Can you work these out from the drawing? Everything is in mm from the part's minimum corner. Round coordinates to 2 decimals unless told otherwise and drop trailing zeros. Loops run counter-clockwise (first coordinate to the right, second up) from the corner with the lowest first, then second, coordinate; pieces in that order, holes last. Notation, with made-up numbers: M -15,-0.5 L 33,-0.5 A24 cw 33,32.5 Z; hole C -14,80.5 d7. An arc over 180 degrees is marked long. Use a Markdown table: item, result.
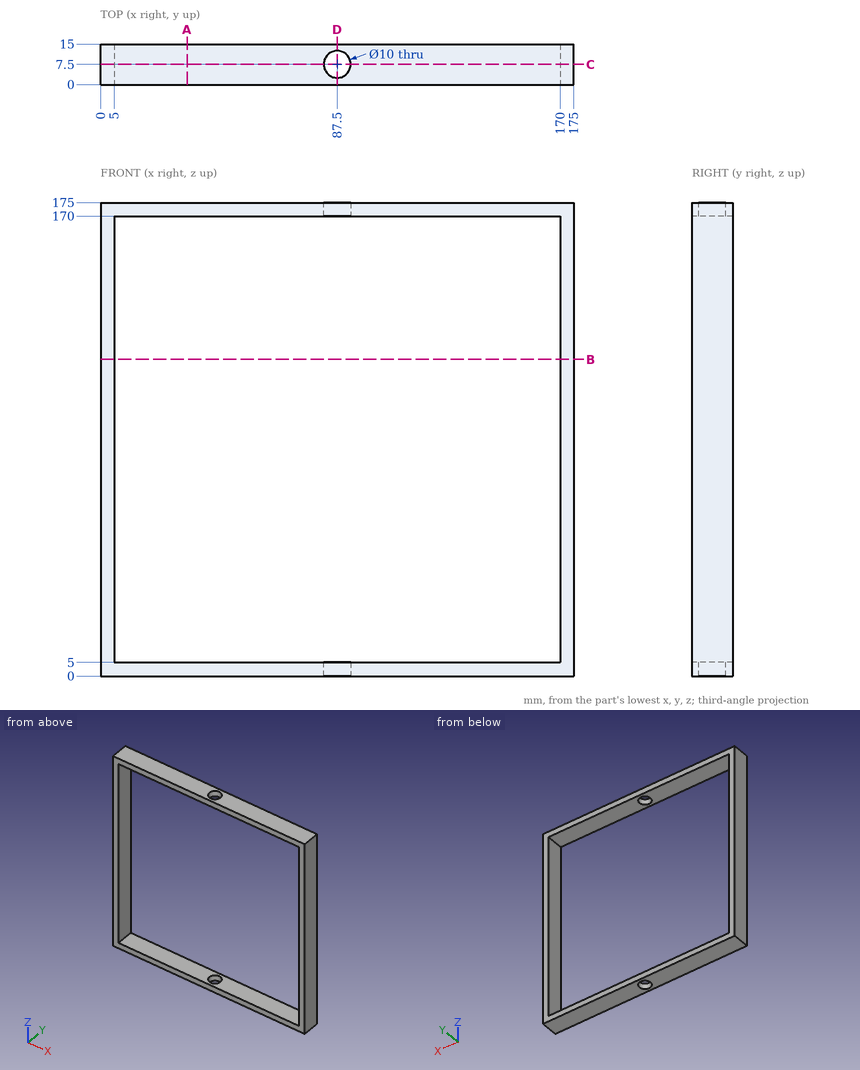
1. Imagine slicing it at A-A, the plane x = 32. Write out the boundary of the cut face in (y, z), then the cut area to 3 significant figures.
Answer sheet:
| item | result |
|---|---|
| outline | M 0,0 L 15,0 L 15,5 L 0,5 Z; M 0,170 L 15,170 L 15,175 L 0,175 Z |
| area | 150 mm2 |
2. Imagine slicing it at D-D, the plane x = 87.5. Write out the boundary of the cut face in (y, z), then the cut area to 3 significant figures.
Answer sheet:
| item | result |
|---|---|
| outline | M 0,0 L 2.5,0 L 2.5,5 L 0,5 Z; M 0,170 L 2.5,170 L 2.5,175 L 0,175 Z; M 12.5,0 L 15,0 L 15,5 L 12.5,5 Z; M 12.5,170 L 15,170 L 15,175 L 12.5,175 Z |
| area | 50.0 mm2 |
3. I need wall thicknesses on probe 1 along Z at (x, y) = (27, 9.25); probe 2 along Y at (x, z) = (87.5, 3.1). Which ranges of each line are inside material? Lowest first, please. Write a range as from..to.
Answer sheet:
| item | result |
|---|---|
| probe 1 | 0..5, 170..175 |
| probe 2 | 0..2.5, 12.5..15 |
4. For pin 1 Ø4.5 at (y, z) = (4, 62.5) entering from -X, with a flat end and sliding along its axis, tell me the tip position at first contact or that it passes through.
Answer sheet:
| item | result |
|---|---|
| pin 1 | x = 0 |
5. Imagine slicing it at B-B, the plane z = 117. Write out the boundary of the cut face in (x, y).
Answer sheet:
| item | result |
|---|---|
| outline | M 0,0 L 5,0 L 5,15 L 0,15 Z; M 170,0 L 175,0 L 175,15 L 170,15 Z |
6. Imagine slicing it at C-C, the plane y = 7.5. Write out the boundary of the cut face in (x, z).
Answer sheet:
| item | result |
|---|---|
| outline | M 0,0 L 82.5,0 L 82.5,5 L 5,5 L 5,170 L 82.5,170 L 82.5,175 L 0,175 Z; M 92.5,0 L 175,0 L 175,175 L 92.5,175 L 92.5,170 L 170,170 L 170,5 L 92.5,5 Z |
